Solid Edge part; units mm, degrees
sketch "Sketch1" plane through (0, 0, 0) normal (0, -1, 0) x (1, 0, 0)
  line L0 (2, 0) -> (3.94, 0)
  line L1 (3.94, 0) -> (3.94, 2)
  line L2 (3.94, 2) -> (3.5, 2)
  line L3 (3.5, 2) -> (3.5, 2.48)
  line L4 (3.5, 2.48) -> (2.69, 2.48)
  line L5 (2.69, 2.48) -> (2.69, 3.38)
  line L6 (2.69, 3.38) -> (2, 3.38)
  line L7 (2, 3.38) -> (2, 0)
  dimension "D1" = 3.94
  dimension "D2" = 2.69
revolve "RevolvedProtrusion1" add sketch "Sketch1" angle 360 about axis through (0, 0, 54) along (0, 0, -1)
The model under review builds one solid part; all positions refer to its coordinate system, in mm. A direction names the side the tool comes from. Round coordinates to 2 decimals unless told otherwise and drop trailing zeros. Order: outer loops, then holes, each group sorted by start corner. A loop starts at its lowest first (then second) coordinate and runs counter-clockwise, first axis right, second up.
Item 1: Add section D-D, the plane y = -2.5. State the section outline as (x, z) points, and give its area (3 significant figures).
Working result:
outline: (-3.05, 0) - (3.05, 0) - (3.05, 2) - (2.45, 2) - (2.45, 2.48) - (0.99, 2.48) - (0.99, 3.38) - (-0.99, 3.38) - (-0.99, 2.48) - (-2.45, 2.48) - (-2.45, 2) - (-3.05, 2) - close
area: 16.3 mm2
Item 2: To check wall thickness, follow probe 1 along X at (y, z) = (0, 2.6); probe 2 along X at (y, z) = (0, 1.85). State the ranges of each line that lie inside material, in increasing order.
Working result:
probe 1: x = -2.69 to -2, 2 to 2.69
probe 2: x = -3.94 to -2, 2 to 3.94
Item 3: Machinability: for faces 4 (the cylindrical face through (-0.583, -2.626, 2.936)), 5 (the flat face through (-2, 1, 3.38)), which of the approach directions +Z, -Z, +X, -X, +Y, -Y give a long, thin tool a straight path to every point of the face, cutting with its end or side? Answer none if there is none.
Working result:
face 4: +Z
face 5: +Z, +X, -X, +Y, -Y
Item 4: Add section A-A, the plane y = 0. State the section outline as (x, z) points, and give its area (3 significant figures).
Working result:
outline: (-3.94, 0) - (-2, 0) - (-2, 3.38) - (-2.69, 3.38) - (-2.69, 2.48) - (-3.5, 2.48) - (-3.5, 2) - (-3.94, 2) - close; (2, 0) - (3.94, 0) - (3.94, 2) - (3.5, 2) - (3.5, 2.48) - (2.69, 2.48) - (2.69, 3.38) - (2, 3.38) - close
area: 10.4 mm2
Item 5: Draft analysis for pull direction Y (two halves, no side actions). For faces 1 (the cylindrical face through (0, 2, 2)), 2 (the cylindrical face through (3.233, -1.341, 2.243)), 3 (the flat face through (-1, 3, 2.48)), state which applies: released by +Y, released by -Y, zero draft, split by the parting line, or undercut.
Working result:
face 1: undercut
face 2: split by the parting line
face 3: zero draft
Item 6: Add section C-C, the plane z = 0.6. State the section outline as (x, y) points.
Working result:
outline: circle Ø7.88 at (0, 0); hole circle Ø4 at (0, 0)
Item 7: For pin 1 (1 mm diameter, centred on x = -1, z = 1.5, fed in from +Y); pin 2 (1 mm diameter, centred on y = 2.5, z = 1.5, fed in from -X), all flat-tipped, find the tip position at first contact; note any pin that passes through.
Working result:
pin 1: stops at y = 3.91
pin 2: stops at x = -3.39
